```python
from build123d import *

# Parameters (mm, degrees)
F1_DEPTH = 6.21
F2_R     = 4.7625
F3_DEPTH = 38.1
F4_SIZE2 = 0.95
F4_SIZE  = 0.95


with BuildPart() as f1:
    # F0 (on Top) → F1 (new body)
    with BuildSketch(Plane.XY):
        Polygon((7.135, 4.119394), (0, 8.238788), (-7.135, 4.119394), (-7.135, -4.119394), (0, -8.238788), (7.135, -4.119394), align=None)
    extrude(amount=-F1_DEPTH)

    # F2 (on face) → F3 (join)
    with BuildSketch(Plane(origin=(0, 0, -6.21), x_dir=(1, 0, 0), z_dir=(0, 0, -1))):
        Circle(F2_R)
    extrude(amount=F3_DEPTH)

    # F4
    f4_edges = [f1.edges().sort_by_distance(p)[0] for p in [
        (-4.7625, 0, -44.31),
    ]]
    chamfer(f4_edges, length=F4_SIZE, length2=F4_SIZE2)

    # F5 (on Right) → F6 (revolve, cut)
    with BuildSketch(Plane.YZ):
        Polygon((8.238788, 0), (7.238788, 0), (8.238788, -1), align=None)
    revolve(axis=Axis((0, 0, -6.21), (0, 0, 1)), mode=Mode.SUBTRACT)


solid = f1.part
```
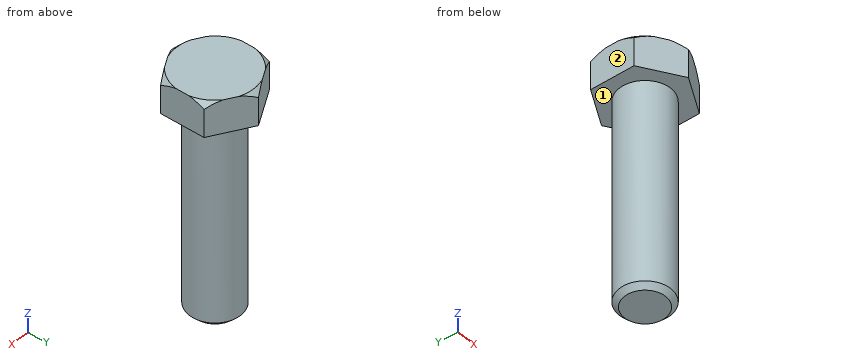
Check sheet for the modelled part. Datum: model origin and axes. Units: mm. Face numbers are marked on the shaded views. A direction names the side the tool comes from. Round coordinates to 2 decimals unless told otherwise and drop trailing zeros. Order: outer loops, then holes, each group sorted by start corner. A loop starts at its lowest first (then second) coordinate and runs counter-clockwise, first axis right, second up. Notation, with made-up numbers: (31, 2.25) - (62, 2.25) arc R9 cw to (62, 6.25) - close; hole circle Ø7 at (-10.75, -17.75). An arc over 180 degrees is marked (long way). Answer as CSV lines item,"result". Start each with the question number.
1) Section check A-A (y = 0). Record the cut outline in (x, z) (1 decimal).
2) Depth check by flat-ended pin: pin 1 (5 mm diameter, centred on x = -0.5, z = -7, fed in from +Y); pin 2 (4 mm diameter, centred on y = 0, z = -9, fed in from +X); pin 3 (1.5 mm diameter, centred on x = 3.5, z = -34, fed in from -Y). Enter the tip coordinate at first touch or a pass-through.
3) Section check C-C (y = -6). Record the cut outline in (x, z), then the cut area to 3 significant figures.
4) Section check B-B (z = -7). Record the cut outline in (x, y) (1 decimal).
5) Scan lines: probe 1 along Z at (x, y) = (-6, 3.75); probe 2 along X at (y, z) = (-2.5, -21); probe 3 along Y at (x, z) = (-2.75, -3). Record each from-to range of solid material in increasing order.
6) Tool access check on the marked faces 1 and 2. Record the directions out of +Z, -Z, +X, -X, +Y, -Y that give a thin tool (end or side, any length) a straight path to the whole face; none if there is none.
Determined:
1,outline,"(-7.1, -6.2) - (-4.8, -6.2) - (-4.8, -43.4) - (-3.8, -44.3) - (3.8, -44.3) - (4.8, -43.4) - (4.8, -6.2) - (7.1, -6.2) - (7.1, 0) - (-7.1, 0) - close"
2,pin 1,"y = 8.24"
2,pin 2,"x = 4.76"
2,pin 3,"y = -3.89"
3,outline,"(-3.88, -6.21) - (3.88, -6.21) - (3.88, 0) - (-3.88, 0) - close"
3,area,"48.2 mm^2"
4,outline,"circle Ø9.5 at (0, 0)"
5,probe 1,"-6.21 to 0"
5,probe 2,"-4.05 to 4.05"
5,probe 3,"-6.65 to 6.65"
6,face 1,"-Z"
6,face 2,"+Z, -Z, -X, +Y, -Y"
